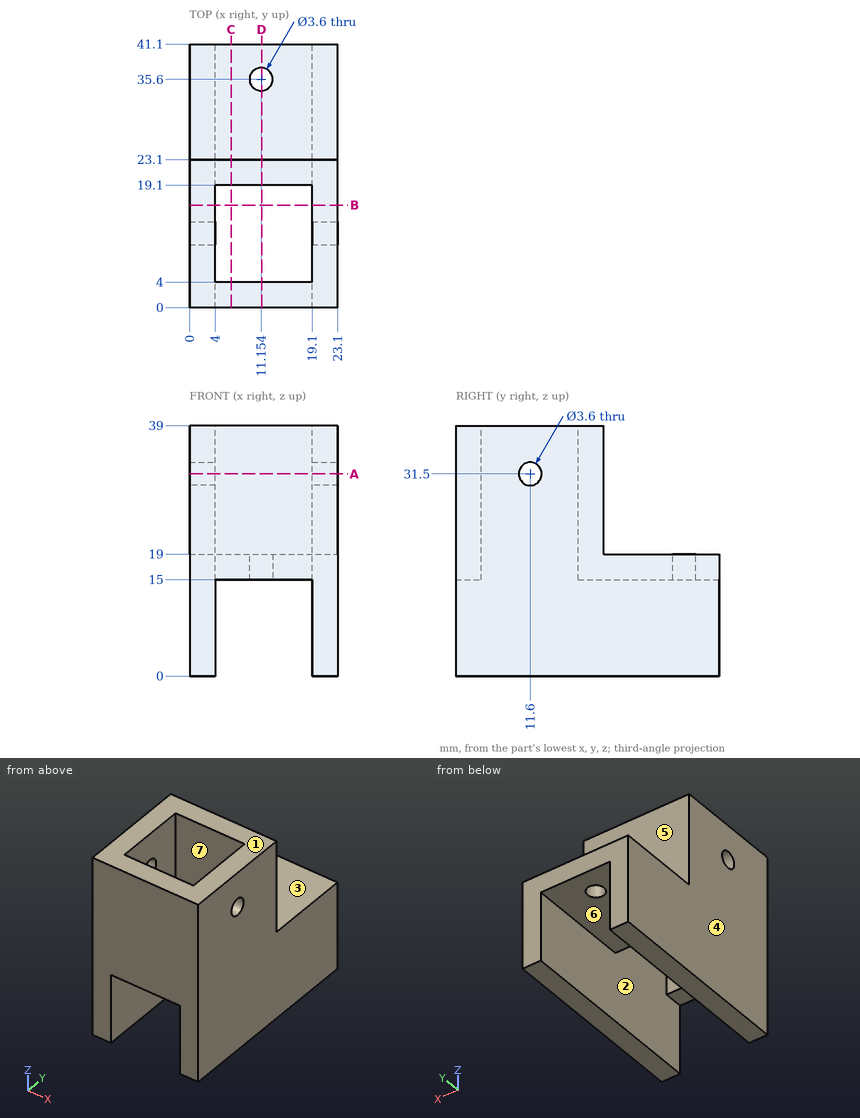
The drawing under review shows one solid part. Ordinate dimensions are in mm from its lowest x, y, z. A direction names the side the tool comes from. Coordinates: 2 decimals unless noted, no trailing zeros. Loops run counter-clockwise (first coordinate to the right, second up) from the corner with the lowest first, then second, coordinate; pieces in that order, holes last. Notation, with made-up numbers: (85.25, -15.75) -> (133.25, -15.75) arc R9 ccw to (133.25, -4.75) -> close; hole circle Ø7 at (-20.75, -15). An arc over 180 degrees is marked (long way). Answer as a JSON object with one key per item and string values.
Q1. Tool access review of the marked faces 1, 2 and 3: name each direction out of +Z, -Z, +X, -X, +Y, -Y from which nothing blocks a thin tool from reaching the whole face with its end or side.
Answer block:
{"face 1": "+Z, +X, -X, +Y, -Y", "face 2": "-Z", "face 3": "+Z, +X, -X, +Y"}
Q2. Take a section at C-C on x = 6.5. Give the boundary of the cut face in (y, z), plus the area to 3 significant figures.
Answer block:
{"outline": "(0, 15) -> (4, 15) -> (4, 39) -> (0, 39) -> close; (19.1, 15) -> (41.1, 15) -> (41.1, 19) -> (23.1, 19) -> (23.1, 39) -> (19.1, 39) -> close", "area": "264 mm^2"}
Q3. The part is to be moulded in two halves that separate along X. For the marked faces 4, 5, 6 and 7, say which applies: +X half, -X half, draft (parallel to the pull), parting line (faces both ways), or undercut.
Answer block:
{"face 4": "-X half", "face 5": "draft", "face 6": "undercut", "face 7": "undercut"}
Q4. To check wall thickness, follow L1, parallel to Y at x = 1.3, z = 31.5; L2, parallel to X at y = 8, z = 5; L3, parallel to Z at x = 21, y = 25.5. State the ranges of each line that lie inside material, in increasing order.
Answer block:
{"L1": "y = 0 to 9.8, 13.4 to 23.1", "L2": "x = 0 to 4, 19.1 to 23.1", "L3": "z = 0 to 19"}
Q5. Take a section at A-A on z = 31.5. Give the boundary of the cut face in (x, y).
Answer block:
{"outline": "(0, 0) -> (23.1, 0) -> (23.1, 9.8) -> (19.1, 9.8) -> (19.1, 4) -> (4, 4) -> (4, 9.8) -> (0, 9.8) -> close; (0, 13.4) -> (4, 13.4) -> (4, 19.1) -> (19.1, 19.1) -> (19.1, 13.4) -> (23.1, 13.4) -> (23.1, 23.1) -> (0, 23.1) -> close"}
Q6. Take a section at D-D on x = 11.25. Give the boundary of the cut face in (y, z).
Answer block:
{"outline": "(0, 15) -> (4, 15) -> (4, 39) -> (0, 39) -> close; (19.1, 15) -> (33.8, 15) -> (33.8, 19) -> (23.1, 19) -> (23.1, 39) -> (19.1, 39) -> close; (37.4, 15) -> (41.1, 15) -> (41.1, 19) -> (37.4, 19) -> close"}
Q7. Clearance check with flat-ended pins moving along their axes: pin 1 Ø4 at (x, y) = (17, 24) entering from -Z; pin 2 Ø3 at (x, y) = (11.15, 35.6) entering from -Z; pin 3 Ø6 at (x, y) = (4, 33.5) entering from +Z. State where each tip first meets the part, or that it passes through.
Answer block:
{"pin 1": "stops at z = 15", "pin 2": "passes through", "pin 3": "stops at z = 19"}
Q8. Take a section at B-B on y = 16. Give the boundary of the cut face in (x, z), plus the area to 3 significant figures.
Answer block:
{"outline": "(0, 0) -> (4, 0) -> (4, 39) -> (0, 39) -> close; (19.1, 0) -> (23.1, 0) -> (23.1, 39) -> (19.1, 39) -> close", "area": "312 mm^2"}
